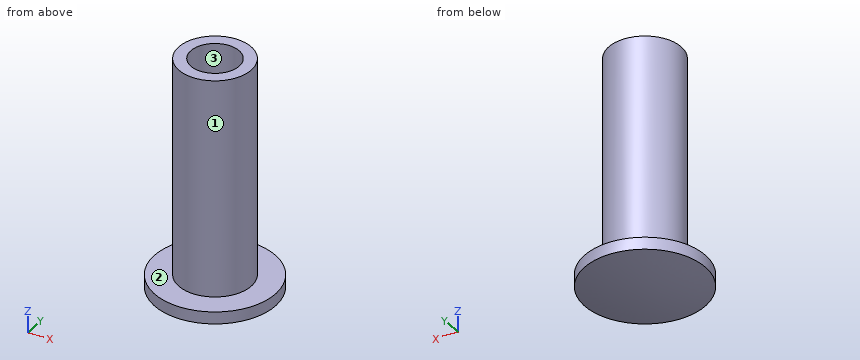
from build123d import *


with BuildPart() as part:
    # Esquisse1 → Révolution1 (revolve)
    with BuildSketch(Plane(origin=(0, 0, 0), x_dir=(0, 0, -1), z_dir=(1, 0, 0))):
        with BuildLine():
            Line((-18, 3), (0, 3))
            Line((0, 3), (0, 5))
            Line((0, 5), (1, 5))
            ThreePointArc((1, 5), (1.357034349, 2.511322427), (1.47640459, 0))
            Line((1.47640459, 0), (0, 0))
            Line((0, 0), (-1.154700538, 2))
            Line((-1.154700538, 2), (-18, 2))
            Line((-18, 2), (-18, 3))
        make_face()
    revolve(axis=Axis((0, 0, 27.655172414), (0, 0, -1)))


solid = part.part
Design review of the part built by this model. Coordinates are the model's own, in mm. Face numbers are marked on the shaded views. Coordinates: 2 decimals unless noted, no trailing zeros. Loops run counter-clockwise (first coordinate to the right, second up) from the corner with the lowest first, then second, coordinate; pieces in that order, holes last. Notation, with made-up numbers: (0, 65) - (32, 65) arc R11 cw to (32, 81) - close; hole circle Ø10 at (37.5, 67.25). An arc over 180 degrees is marked (long way). Use CSV: the item, a comma, the result in double quotes. Start each with the question number.
1. Add section B-B on x = -2.5. Give the boundary of the cut face in (y, z), plus the area to 3 significant figures.
2. Add section A-A on z = 10.75. Give the boundary of the cut face in (x, y), plus the area to 3 significant figures.
3. To check wall thickness, follow probe 1 along X at (y, z) = (0, 9); probe 2 along Y at (x, z) = (-0.25, 10.25); probe 3 along Y at (x, z) = (-1.5, 10.75). State the ranges of each line that lie inside material, in increasing order.
4. Add section C-C on x = 4.5. Give the boundary of the cut face in (y, z).
5. Mouldability with a two-part tool opening along Y and no side actions: class the marked faces 1, 2 and 3 as released by +Y, released by -Y, zero draft, split by the parting line, or undercut.
6. Clearance check with flat-ended pins moving along their axes: pin 1 (4 mm diameter, centred on y = 2, z = 9.5, fed in from -X); pin 2 (4 mm diameter, centred on x = -4, z = 6, fed in from -Y); pin 3 (1.5 mm diameter, centred on x = 2, y = -0.5, fed in from -Z). State where each tip first meets the part, or that it passes through.
Resolved:
1,outline,"(-4.33, -1) arc R26.36 ccw to (4.33, -1) - (4.33, 0) - (1.66, 0) - (1.66, 18) - (-1.66, 18) - (-1.66, 0) - (-4.33, 0) - close"
1,area,"70.4 mm2"
2,outline,"circle Ø6 at (0, 0); hole circle Ø4 at (0, 0)"
2,area,"15.7 mm2"
3,probe 1,"-3 to -2, 2 to 3"
3,probe 2,"-2.99 to -1.98, 1.98 to 2.99"
3,probe 3,"-2.6 to -1.32, 1.32 to 2.6"
4,outline,"(-2.18, -1) arc R26.09 ccw to (2.18, -1) - (2.18, 0) - (-2.18, 0) - close"
5,face 1,"split by the parting line"
5,face 2,"zero draft"
5,face 3,"undercut"
6,pin 1,"x = -3"
6,pin 2,"y = -2.24"
6,pin 3,"z = -1.44"
